from build123d import *

# Parameters (mm, degrees)
SKETCH2_R           = 8
SKETCH2_R_2         = 1.4
BOSS_EXTRUDE1_DEPTH = 3
FILLET1_R           = 1


with BuildPart() as part:
    # Sketch2 → Boss-Extrude1 (new body)
    with BuildSketch(Plane.XY):
        with BuildLine():
            ThreePointArc((2.368452446, -25.752812678), (1.754211193, -30.008558133), (2.368452446, -34.264303588))
            ThreePointArc((2.368452446, -34.264303588), (2.650810328, -37.36580095), (1.727482394, -40.34010379))
            ThreePointArc((1.727482394, -40.34010379), (2.329337459, -44.483431868), (6.472665536, -45.085286933))
            ThreePointArc((6.472665536, -45.085286933), (9.446968377, -44.161958999), (12.548465738, -44.444316881))
            ThreePointArc((12.548465738, -44.444316881), (16.804211193, -45.058558133), (21.059956649, -44.444316881))
            ThreePointArc((21.059956649, -44.444316881), (24.16145401, -44.161958999), (27.135756851, -45.085286933))
            ThreePointArc((27.135756851, -45.085286933), (31.279084928, -44.483431868), (31.880939993, -40.34010379))
            ThreePointArc((31.880939993, -40.34010379), (30.957612059, -37.36580095), (31.239969941, -34.264303588))
            ThreePointArc((31.239969941, -34.264303588), (31.854211193, -30.008558133), (31.239969941, -25.752812678))
            ThreePointArc((31.239969941, -25.752812678), (30.957612059, -22.651315316), (31.880939993, -19.677012476))
            ThreePointArc((31.880939993, -19.677012476), (31.279084928, -15.533684399), (27.135756851, -14.931829334))
            ThreePointArc((27.135756851, -14.931829334), (24.16145401, -15.855157268), (21.059956649, -15.572799386))
            ThreePointArc((21.059956649, -15.572799386), (16.804211193, -14.958558133), (12.548465738, -15.572799386))
            ThreePointArc((12.548465738, -15.572799386), (9.446968377, -15.855157268), (6.472665536, -14.931829334))
            ThreePointArc((6.472665536, -14.931829334), (2.329337459, -15.533684399), (1.727482394, -19.677012476))
            ThreePointArc((1.727482394, -19.677012476), (2.650810328, -22.651315316), (2.368452446, -25.752812678))
        make_face()
        with Locations((16.804211193, -30.008558133)):
            Circle(SKETCH2_R, mode=Mode.SUBTRACT)
        with Locations((4.804211193, -18.008558133)):
            Circle(SKETCH2_R_2, mode=Mode.SUBTRACT)
        with Locations((28.804211193, -18.008558133)):
            Circle(SKETCH2_R_2, mode=Mode.SUBTRACT)
        with Locations((28.804211193, -42.008558133)):
            Circle(SKETCH2_R_2, mode=Mode.SUBTRACT)
        with Locations((4.804211193, -42.008558133)):
            Circle(SKETCH2_R_2, mode=Mode.SUBTRACT)
    extrude(amount=BOSS_EXTRUDE1_DEPTH)

    # Fillet1
    fillet1_edges = [part.edges().sort_by_distance(p)[0] for p in [
        (2.329337459, -15.533684399, 0),
        (9.446968377, -15.855157268, 0),
        (16.804211193, -14.958558133, 0),
        (24.16145401, -15.855157268, 0),
        (31.279084928, -15.533684399, 0),
        (30.957612059, -22.651315316, 0),
        (31.854211193, -30.008558133, 0),
        (30.957612059, -37.36580095, 0),
        (31.279084928, -44.483431868, 0),
        (24.16145401, -44.161958999, 0),
        (16.804211193, -45.058558133, 0),
        (9.446968377, -44.161958999, 0),
        (2.329337459, -44.483431868, 0),
        (2.650810328, -37.36580095, 0),
        (1.754211193, -30.008558133, 0),
        (2.650810328, -22.651315316, 0),
        (8.804211193, -30.008558133, 0),
    ]]
    fillet(fillet1_edges, radius=FILLET1_R)


solid = part.part
The listing builds one solid part. Answer for the finished solid, in the listing's coordinates (mm). Coordinates: 2 decimals unless noted, no trailing zeros. Order: outer loops, then holes, each group sorted by start corner. A loop starts at its lowest first (then second) coordinate and runs counter-clockwise, first axis right, second up.
Q1. A cutting plane is placed at B-B, the plane x = 4.5. State how many separate pieces and enclosed holes the cut face has, and give its area (3 significant figures).
Q2. Consider line 1 (Y direction, x = 29, z = 1.45); line 2 (X direction, y = -30, z = 2.6); line 3 (Y direction, x = 5, z = 0.5). Determine where each line is inside the solid, lowest interval first.
Q3. A cutting plane is placed at A-A, the plane z = 2. Write down the section's boundary in (x, y).
Q4. For a pull along Y with two mould halves and no side action, classify faces 1 (the face through (9.403, -44.167, 1.986)), 2 (the face through (31.854, -30.069, 1.986)), 3 (the face through (16.86, -14.96, 1.99)) as pulls with the +Y half, pulls with the -Y half, needs draft (parallel to the pull), parting line crosses it, or undercut.
Answers follow:
1. separate pieces: 3
1. enclosed holes: 0
1. area: 76.1 mm2
2. line 1: y = -45.5 to -43.39, -40.62 to -19.39, -16.62 to -14.51
2. line 2: x = 1.75 to 8.8, 24.8 to 31.85
2. line 3: y = -45.37 to -43.39, -40.62 to -19.39, -16.62 to -14.65
3. outline: (1.73, -40.34) arc R3.5 ccw to (6.47, -45.09) arc R8 cw to (12.55, -44.44) arc R15.05 ccw to (21.06, -44.44) arc R8 cw to (27.14, -45.09) arc R3.5 ccw to (31.88, -40.34) arc R8 cw to (31.24, -34.26) arc R15.05 ccw to (31.24, -25.75) arc R8 cw to (31.88, -19.68) arc R3.5 ccw to (27.14, -14.93) arc R8 cw to (21.06, -15.57) arc R15.05 ccw to (12.55, -15.57) arc R8 cw to (6.47, -14.93) arc R3.5 ccw to (1.73, -19.68) arc R8 cw to (2.37, -25.75) arc R15.05 ccw to (2.37, -34.26) arc R8 cw to start; hole circle Ø2.8 at (4.8, -42.01); hole circle Ø2.8 at (4.8, -18.01); hole circle Ø16 at (16.8, -30.01); hole circle Ø2.8 at (28.8, -42.01); hole circle Ø2.8 at (28.8, -18.01)
4. face 1: pulls with the -Y half
4. face 2: undercut
4. face 3: pulls with the +Y half
